from build123d import *

# Parameters (mm, degrees)
SKETCH1_R                   = 62
BOSS_EXTRUDE1_DEPTH         = 15
SKETCH2_R                   = 2
CUT_EXTRUDE1_DEPTH          = 15
CIRPATTERN1_COUNT           = 2
CIRPATTERN1_ANGLE           = 60
CIRPATTERN2_COUNT           = 2
CIRPATTERN2_COPY_1_SKETCH_R = 2
CIRPATTERN2_COPY_1_DEPTH    = 15
SKETCH3_R                   = 6.1
CUT_EXTRUDE2_DEPTH          = 15


with BuildPart() as part:
    # Sketch1 → Boss-Extrude1 (new body)
    with BuildSketch(Plane.XY):
        Circle(SKETCH1_R)
    extrude(amount=BOSS_EXTRUDE1_DEPTH)

    # Sketch2 → Cut-Extrude1 (cut)
    with BuildSketch(Plane.XY.offset(15)):
        with Locations((0, 49.5)):
            Circle(SKETCH2_R)
    cut_extrude1 = extrude(amount=-CUT_EXTRUDE1_DEPTH, mode=Mode.SUBTRACT)

    # CirPattern1: Cut-Extrude1 ×2 about axis
    cirpattern1_axis = Axis((0, 0, 15), (0, 0, -1))
    for i in range(1, CIRPATTERN1_COUNT):
        add(cut_extrude1.rotate(cirpattern1_axis, i * CIRPATTERN1_ANGLE / (CIRPATTERN1_COUNT - 1)), mode=Mode.SUBTRACT)

    # CirPattern2: Cut-Extrude1 ×2 about axis
    cirpattern2_axis = Axis((0, 0, 0), (0, 0, 1))
    for i in range(1, CIRPATTERN2_COUNT):
        add(cut_extrude1.rotate(cirpattern2_axis, i * 360 / CIRPATTERN2_COUNT), mode=Mode.SUBTRACT)

    # CirPattern2 copy 1 sketch → CirPattern2 copy 1 (cut)
    with BuildSketch(Plane(origin=(0, 0, 15), x_dir=(-0.49999999999999767, 0.86602540378444, 0), z_dir=(0, 0, 1))):
        with Locations((0, 49.5)):
            Circle(CIRPATTERN2_COPY_1_SKETCH_R)
    extrude(amount=-CIRPATTERN2_COPY_1_DEPTH, mode=Mode.SUBTRACT)

    # Sketch3 → Cut-Extrude2 (cut)
    with BuildSketch(Plane.XY.offset(15)):
        Circle(SKETCH3_R)
    extrude(amount=-CUT_EXTRUDE2_DEPTH, mode=Mode.SUBTRACT)


solid = part.part
Build history of the part. All positions in model axes, mm. Coordinates: 2 decimals unless noted, no trailing zeros. Write each loop counter-clockwise with the first axis right and the second up, starting at its lowest first coordinate (ties: lowest second). Pieces come first, ordered by that corner, then holes. Notation, with made-up numbers: (14, 43) -> (51, 43) arc R22 cw to (51, 68) -> close; hole circle Ø8 at (-13.75, 19.5). An arc over 180 degrees is marked (long way). Use CSV: the item, a comma, the result in double quotes. Start each with the question number.
Q1. Cut at C-C, the plane y = 24.5. List the corners of the cut face in (x, z).
Q2. Cut at D-D, the plane x = -14. List the corners of the cut face in (y, z).
Q3. Pull direction X, two halves, no side cores. Call faces 1 (the flat face through (-1, -13, 0)), 2 (the cylindrical face through (-6.094, 0.268, 7.605)), 3 (the cylindrical face through (-41.793, -23.064, 7.605)), 4 (the cylindrical face through (-8.071, 61.472, 7.395)): released by +X, released by -X, zero draft, split by the parting line, or undercut.
Q4. Cut at A-A, the plane y = 0. List the corners of the cut face in (x, z).
Q5. Drill centre lines: probe 1 along Y at (x, z) = (0, 3); probe 2 along Y at (x, z) = (4, 5.5); probe 3 along Y at (x, z) = (23, 5). Where is each one in solid material? Low to high.
Q6. Cut at B-B, the plane z = 2. List the corners of the cut face in (x, y), then the cut area to 3 significant figures.
Q7. Flat gauge pins, fed straight in: pin 1 Ø19.5 at (x, y) = (0, 0) entering from -Z; pin 2 Ø1 at (y, z) = (-18.5, 11) entering from -X; pin 3 Ø1.5 at (y, z) = (38, 10) entering from +X; pin 4 Ø4 at (x, z) = (45, 5) entering from +Y. Where does each tip first touch, or does it go through?
Checked values:
1,outline,"(-56.95, 0) -> (40.88, 0) -> (40.88, 15) -> (-56.95, 15) -> close; (44.85, 0) -> (56.95, 0) -> (56.95, 15) -> (44.85, 15) -> close"
2,outline,"(-60.4, 0) -> (60.4, 0) -> (60.4, 15) -> (-60.4, 15) -> close"
3,face 1,"zero draft"
3,face 2,"undercut"
3,face 3,"undercut"
3,face 4,"split by the parting line"
4,outline,"(-62, 0) -> (-6.1, 0) -> (-6.1, 15) -> (-62, 15) -> close; (6.1, 0) -> (62, 0) -> (62, 15) -> (6.1, 15) -> close"
5,probe 1,"y = -62 to -51.5, -47.5 to -6.1, 6.1 to 47.5, 51.5 to 62"
5,probe 2,"y = -61.87 to -4.61, 4.61 to 61.87"
5,probe 3,"y = -57.58 to 57.58"
6,outline,"circle Ø124 at (0, 0); hole circle Ø4 at (-42.87, -24.75); hole circle Ø12.2 at (0, 0); hole circle Ø4 at (0, -49.5); hole circle Ø4 at (0, 49.5); hole circle Ø4 at (42.87, 24.75)"
6,area,"11,900 mm²"
7,pin 1,"stops at z = 0"
7,pin 2,"stops at x = -59.33"
7,pin 3,"stops at x = 49.56"
7,pin 4,"stops at y = 44.67"
